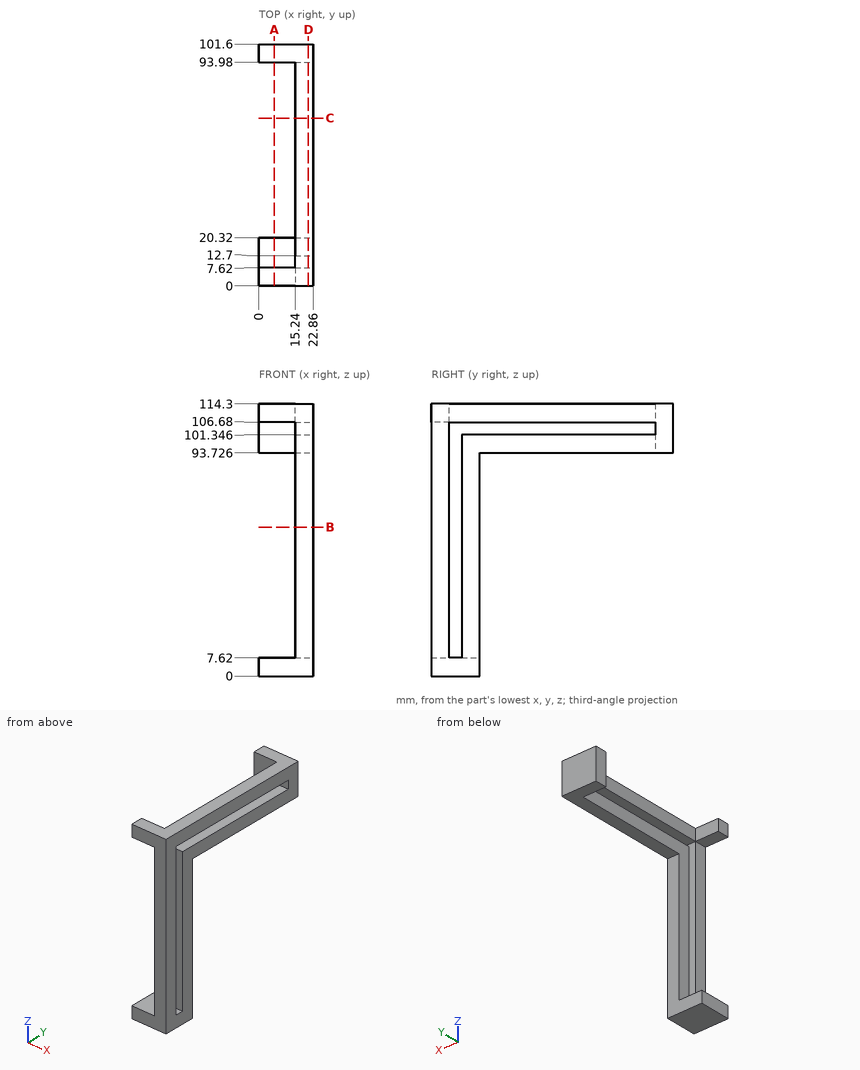
The drawing under review shows one solid part. Ordinate dimensions are in mm from its lowest x, y, z. Coordinates: 2 decimals unless noted, no trailing zeros. Order: outer loops, then holes, each group sorted by start corner. A loop starts at its lowest first (then second) coordinate and runs counter-clockwise, first axis right, second up. Notation, with made-up numbers: (-38, 87) -> (-16, 87) arc R14 cw to (-16, 92) -> close; hole circle Ø7 at (7, 38.25). An arc over 180 degrees is marked (long way). Return JSON: item names as keys, results as strings.
1. For pin 1 Ø4 at (x, y) = (18.5, 59.5) entering from -Z; pin 2 Ø4 at (y, z) = (55, 110.5) entering from -X; pin 3 Ø6 at (x, z) = (18.5, 57.5) entering from -Y; pin 4 Ø2.5 at (x, z) = (21, 52) entering from +Y, all flat-tipped, find the tip position at first contact; note any pin that passes through.
Answer block:
{"pin 1": "z = 93.73", "pin 2": "x = 15.24", "pin 3": "y = 0", "pin 4": "y = 20.32"}
2. We need section D-D on x = 20.75. Write out the cut boundary in (y, z), and give its area (3 significant figures).
Answer block:
{"outline": "(0, 0) -> (20.32, 0) -> (20.32, 93.73) -> (101.6, 93.73) -> (101.6, 114.3) -> (0, 114.3) -> close; hole (7.62, 7.62) -> (12.7, 7.62) -> (12.7, 101.35) -> (93.98, 101.35) -> (93.98, 106.68) -> (7.62, 106.68) -> close", "area": "3,060 mm²"}
3. We need section A-A on x = 6.5. Write out the cut boundary in (y, z).
Answer block:
{"outline": "(0, 0) -> (20.32, 0) -> (20.32, 7.62) -> (0, 7.62) -> close; (0, 106.68) -> (7.62, 106.68) -> (7.62, 114.3) -> (0, 114.3) -> close; (93.98, 93.73) -> (101.6, 93.73) -> (101.6, 114.3) -> (93.98, 114.3) -> close"}
4. We need section C-C on y = 70.5. Write out the cut boundary in (x, z).
Answer block:
{"outline": "(15.24, 93.73) -> (22.86, 93.73) -> (22.86, 101.35) -> (15.24, 101.35) -> close; (15.24, 106.68) -> (22.86, 106.68) -> (22.86, 114.3) -> (15.24, 114.3) -> close"}
5. We need section B-B on z = 62.5. Write out the cut boundary in (x, y), and give its area (3 significant figures).
Answer block:
{"outline": "(15.24, 0) -> (22.86, 0) -> (22.86, 7.62) -> (15.24, 7.62) -> close; (15.24, 12.7) -> (22.86, 12.7) -> (22.86, 20.32) -> (15.24, 20.32) -> close", "area": "116 mm²"}
6. For line 1 (Z direction, x = 19.5, y = 61.5); line 2 (Z direction, x = 3.5, y = 4.5); line 3 (Y direction, x = 20.25, z = 12), list the stretches that pass through material, from the lowest coordinate up. Write a range as from..to.
Answer block:
{"line 1": "93.73..101.35, 106.68..114.3", "line 2": "0..7.62, 106.68..114.3", "line 3": "0..7.62, 12.7..20.32"}
